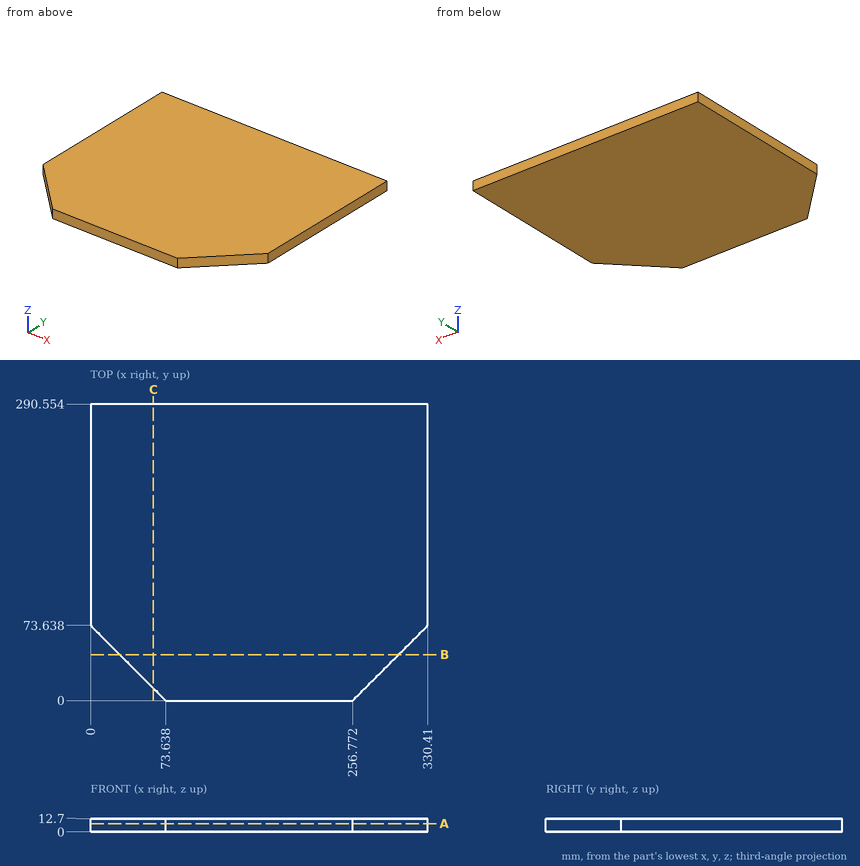
For this review, use the dimensioned drawing (mm, ordinates from the lowest corner) and the shaded views. Round coordinates to 2 decimals unless told otherwise and drop trailing zeros. Loops run counter-clockwise (first coordinate to the right, second up) from the corner with the lowest first, then second, coordinate; pieces in that order, holes last. Notation, with made-up numbers: (58, -10.5) -> (88, -10.5) arc R25 ccw to (88, 25.5) -> close; hole circle Ø1 at (62, 38.5). An arc over 180 degrees is marked (long way). Write item = value, one per line. Start each with the question number.
Item 1: Take a section at B-B on y = 45. Give the boundary of the cut face in (x, z), plus the area to 3 significant figures.
Item 2: Take a section at A-A on z = 7.75. Give the boundary of the cut face in (x, y), plus the area to 3 significant figures.
Item 3: Take a section at C-C on x = 61.5. Give the boundary of the cut face in (y, z).
Item 4: To check wall thickness, follow L1, parallel to Y at x = 60, z = 3.25 (1 decimal); L2, parallel to X at y = 49, z = 8.5; L3, parallel to X at y = 29.5, z = 5.75. State the ranges of each line that lie inside material, in increasing order.
Result:
q1.outline = (28.64, 0) -> (301.77, 0) -> (301.77, 12.7) -> (28.64, 12.7) -> close
q1.area = 3,470 mm²
q2.outline = (0, 73.64) -> (73.64, 0) -> (256.77, 0) -> (330.41, 73.64) -> (330.41, 290.55) -> (0, 290.55) -> close
q2.area = 90,600 mm²
q3.outline = (12.14, 0) -> (290.55, 0) -> (290.55, 12.7) -> (12.14, 12.7) -> close
q4.L1 = 13.6 to 290.6
q4.L2 = 24.64 to 305.77
q4.L3 = 44.14 to 286.27
